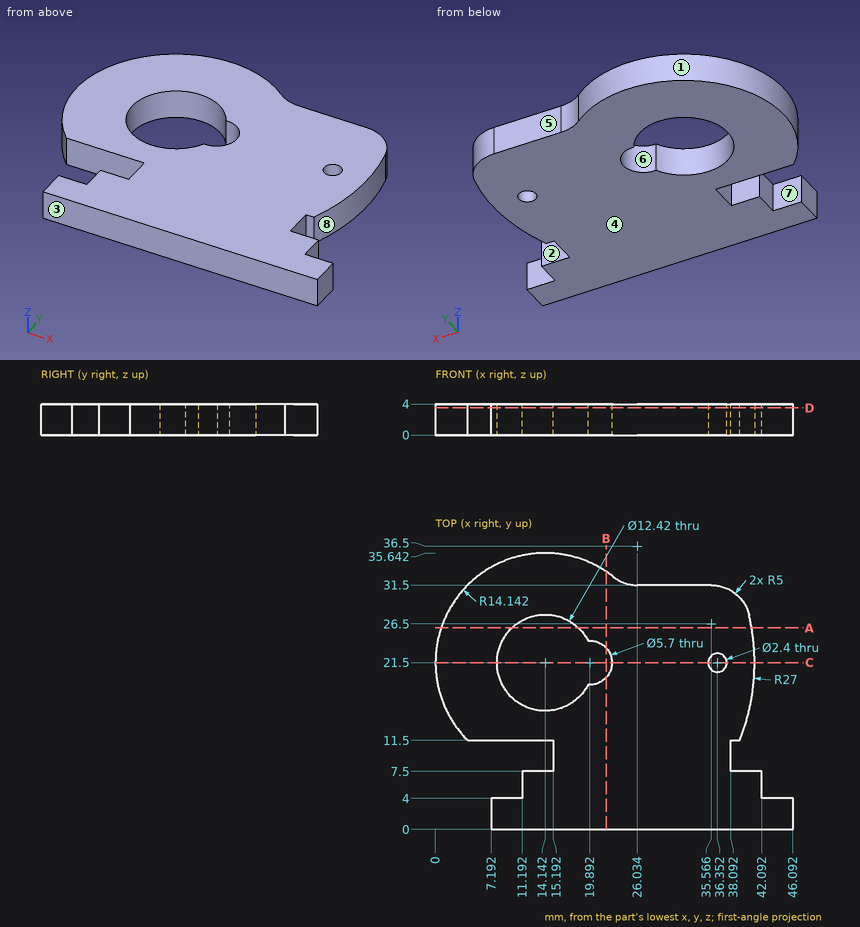
Design review of the part shown in the three views and the two pictorial views. Dimensions are in mm from the part's minimum x, y and z. A direction names the side the tool comes from. Give positions to 0.01 mm unless a question says otherwise; leave off trailing zeros. Loops run counter-clockwise (first coordinate to the right, second up) from the corner with the lowest first, then second, coordinate; pieces in that order, holes last. Notation, with made-up numbers: (63, -10) -> (117, -10) arc R7 cw to (117, 3) -> close; hole circle Ø6 at (21, -1.5). An arc over 180 degrees is marked (long way). One line per item, written item: value.
Q1. Draft analysis for pull direction Y (two halves, no side actions). For the marked faces 1, 2 and 3, state which applies: pulls with the +Y half, pulls with the -Y half, needs draft (parallel to the pull), parting line crosses it, or undercut.
Numbers:
face 1: parting line crosses it
face 2: undercut
face 3: pulls with the -Y half
Q2. We need section B-B on x = 22. Give the boundary of the cut face in (y, z), and give its area (3 significant figures).
Numbers:
outline: (0, 0) -> (19.58, 0) -> (19.58, 4) -> (0, 4) -> close; (23.42, 0) -> (33.26, 0) -> (33.26, 4) -> (23.42, 4) -> close
area: 118 mm^2
Q3. We need section C-C on y = 21.5. Give the boundary of the cut face in (x, z).
Numbers:
outline: (0, 0) -> (7.93, 0) -> (7.93, 4) -> (0, 4) -> close; (22.74, 0) -> (35.15, 0) -> (35.15, 4) -> (22.74, 4) -> close; (37.55, 0) -> (41.14, 0) -> (41.14, 4) -> (37.55, 4) -> close
Q4. We need section A-A on y = 26. Give the boundary of the cut face in (x, z) (1 decimal), and give its area (3 significant figures).
Numbers:
outline: (0.7, 0) -> (9.9, 0) -> (9.9, 4) -> (0.7, 4) -> close; (18.4, 0) -> (40.8, 0) -> (40.8, 4) -> (18.4, 4) -> close
area: 126 mm^2
Q5. Machinability: for the marked faces 4, 5, 6, 7 and 8, which of the approach directions +Z, -Z, +X, -X, +Y, -Y give a long, thin tool a straight path to every point of the face, cutting with its end or side? Answer none if there is none.
Numbers:
face 4: -Z, +X, -X, +Y, -Y
face 5: +Z, -Z, +X, +Y
face 6: +Z, -Z
face 7: +Z, -Z, -X
face 8: +Z, -Z, +X
Q6. For pin 1 Ø1.2 at (y, z) = (3, 2) entering from -X; pin 2 Ø1.2 at (x, z) = (32.5, 2) entering from +Y; pin 3 Ø16 at (x, y) = (14.14, 21.5) entering from +Z; pin 4 Ø2 at (x, z) = (44.5, 2.5) entering from +Y, all flat-tipped, find the tip position at first contact; note any pin that passes through.
Numbers:
pin 1: stops at x = 7.19
pin 2: stops at y = 31.5
pin 3: stops at z = 4
pin 4: stops at y = 4
Q7. For L1, parallel to Y at x = 13.5, z = 0.65; L2, parallel to Y at x = 44, z = 0.25; L3, parallel to Y at x = 10, z = 2.8 (1 decimal), list the stretches that pass through material, from the lowest coordinate up.
Numbers:
L1: y = 0 to 7.5, 11.5 to 15.32, 27.68 to 35.63
L2: y = 0 to 4
L3: y = 0 to 4, 11.5 to 16.9, 26.1 to 35
Q8. We need section D-D on z = 3.5. Give the number of separate pieces and of enclosed holes in the cut face, and give its area (3 significant figures).
Numbers:
separate pieces: 1
enclosed holes: 2
area: 1,060 mm^2
